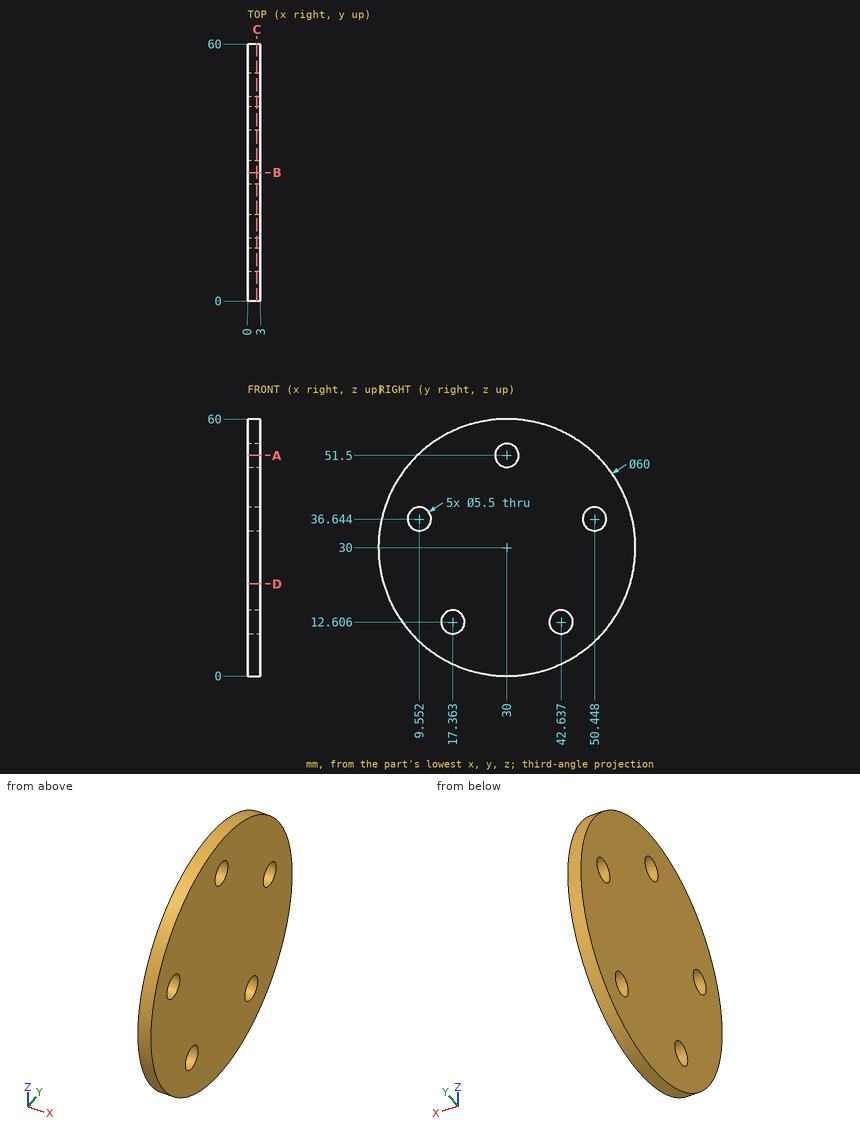
Part print with two shaded views. Sizes in mm from the minimum x, y, z corner. Round coordinates to 2 decimals unless told otherwise and drop trailing zeros. Write each loop counter-clockwise with the first axis right and the second up, starting at its lowest first coordinate (ties: lowest second). Pieces come first, ordered by that corner, then holes. Notation, with made-up numbers: M 34.5,62.5 L 42.5,62.5 A20 ccw 42.5,71.5 Z; hole C 55.5,45.5 d2. An arc over 180 degrees is marked long. Put each result on its own line as item: value. Start each with the question number.
1) Saw through at B-B, the plane y = 30. Write the cut outline in (x, z).
2) Drill centre lines: probe 1 along Y at (x, z) = (1.45, 11) (1 decimal); probe 2 along Y at (x, z) = (1, 15) (1 decimal); probe 3 along Z at (x, y) = (1.55, 43). Where is each one in solid material? Low to high. Write a range as [from, to].
3) Saw through at A-A, the plane z = 51.5. Write the cut outline in (x, y).
4) Saw through at D-D, the plane z = 21.5. Write the cut outline in (x, y).
5) Pin check, flat tips, straight feed: pin 1 Ø3.5 at (y, z) = (42.64, 12.61) entering from -X (3 decimals); pin 2 Ø1 at (x, y) = (2, 36) entering from +Z; pin 3 Ø1 at (x, y) = (1.5, 32) entering from +Z. Stop position of each tip, or through.
6) Saw through at C-C, the plane x = 2.2. Write the cut outline in (y, z), and give its area (3 significant figures).
Resolved:
1. outline: M 0,0 L 3,0 L 3,48.75 L 0,48.75 Z; M 0,54.25 L 3,54.25 L 3,60 L 0,60 Z
2. probe 1: [6.8, 15.1], [19.6, 40.4], [44.9, 53.2]
2. probe 2: [4, 16], [18.7, 41.3], [44, 56]
2. probe 3: [2.96, 9.88], [15.33, 57.04]
3. outline: M 0,9.08 L 3,9.08 L 3,27.25 L 0,27.25 Z; M 0,32.75 L 3,32.75 L 3,50.92 L 0,50.92 Z
4. outline: M 0,1.23 L 3,1.23 L 3,58.77 L 0,58.77 Z
5. pin 1: through
5. pin 2: z = 59.49
5. pin 3: z = 59.96
6. outline: C 30,30 d60; hole C 9.55,36.64 d5.5; hole C 17.36,12.61 d5.5; hole C 30,51.5 d5.5; hole C 42.64,12.61 d5.5; hole C 50.45,36.64 d5.5
6. area: 2,710 mm²
